Can you work these out from the model? Positions are in its coordinate system, mm. Face numbers are marked on the shaded views. Give positions to 0.01 mm unless a question says otherwise; leave off trailing zeros. Loops run counter-clockwise (first coordinate to the right, second up) from the corner with the lowest first, then second, coordinate; pieces in that order, holes last. Notation, with made-up numbers: (52, 55) -> (88, 55) arc R27 cw to (88, 74) -> close; hole circle Ø3 at (49.5, 34). An arc over 180 degrees is marked (long way). One line per question, with ' | ' between items.
from build123d import *

# Parameters (mm, degrees)
SKETCH1_R           = 39.37
SKETCH1_R_2         = 38.1
BOSS_EXTRUDE1_DEPTH = 685.8
SKETCH2_R           = 1.692869147
CUT_EXTRUDE1_DEPTH  = 61.4
CIRPATTERN3_COUNT   = 3
CUT_EXTRUDE2_DEPTH  = 72.4


with BuildPart() as part:
    # Sketch1 → Boss-Extrude1 (new body)
    with BuildSketch(Plane(origin=(0, 0, 0), x_dir=(1, 0, 0), z_dir=(0, 1, 0))):
        with Locations(Location((0, 0, 0), (0, 0, 270))):
            Circle(SKETCH1_R)
        with Locations(Location((0, 0, 0), (0, 0, 270))):
            Circle(SKETCH1_R_2, mode=Mode.SUBTRACT)
    extrude(amount=BOSS_EXTRUDE1_DEPTH)

    # Sketch2 → Cut-Extrude1 (cut)
    with BuildSketch(Plane.XY):
        with Locations(Location((0, 3.287142885, 0), (0, 0, 90))):
            Circle(SKETCH2_R)
    cut_extrude1 = extrude(amount=-CUT_EXTRUDE1_DEPTH, mode=Mode.SUBTRACT)

    # CirPattern3: Cut-Extrude1 ×3 about axis
    cirpattern3_axis = Axis((0, 0, 0), (0, -1, 0))
    for i in range(1, CIRPATTERN3_COUNT):
        add(cut_extrude1.rotate(cirpattern3_axis, i * 360 / CIRPATTERN3_COUNT), mode=Mode.SUBTRACT)

    # Sketch3 → Cut-Extrude2 (cut)
    with BuildSketch(Plane(origin=(0, 0, 0), x_dir=(0, 0, -1), z_dir=(1, 0, 0))):
        Polygon((-39.37, 513.990392655), (39.37, 513.990392655), (39.37, 282.655028446), (39.37, 269.955028446), (39.37, 263.605028446), (-39.37, 263.605028446), (-39.37, 269.955028446), (-39.37, 276.305028446), (-39.37, 282.655028446), align=None)
    extrude(amount=CUT_EXTRUDE2_DEPTH, mode=Mode.SUBTRACT)


solid = part.part
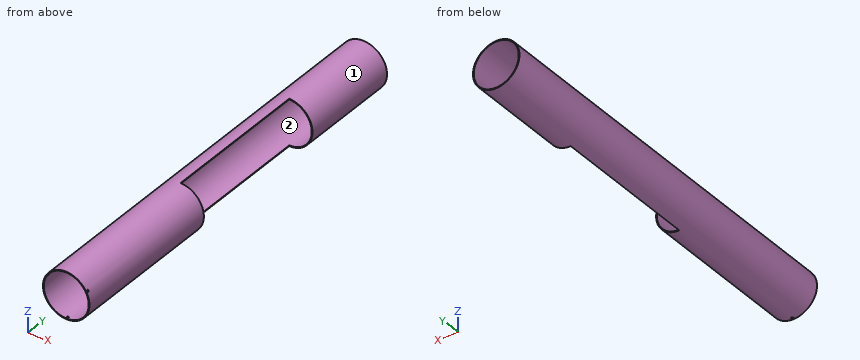
Q1. If we section it at A-A (z = 0): Write out the boundary of the cut face in (x, y), plus the area to 3 significant figures.
Entries:
outline: (-39.37, 0) -> (-38.1, 0) -> (-38.1, 685.8) -> (-39.37, 685.8) -> close; (38.1, 0) -> (39.37, 0) -> (39.37, 263.61) -> (38.1, 263.61) -> close; (38.1, 513.99) -> (39.37, 513.99) -> (39.37, 685.8) -> (38.1, 685.8) -> close | area: 1,420 mm²
Q2. For pin 1 Ø5 at (x, z) = (18.5, 28.5) entering from -Y; pin 2 Ø1.4 at (y, z) = (408, 38.5) entering from +X; pin 3 Ø3 at (y, z) = (507.5, 28.5) entering from -X; pin 4 Ø2 at (x, y) = (0, 3.29) entering from -Z, each with a flat end and sliding along its axis, tell me the tip position at first contact or that it passes through.
Entries:
pin 1: through | pin 2: x = 0 | pin 3: x = -28.65 | pin 4: z = 38.09
Q3. If we section it at D-D (y = 247): Write out the boundary of the cut face in (x, z), plus the area to 3 significant figures.
Entries:
outline: circle Ø78.74 at (0, 0); hole circle Ø76.2 at (0, 0) | area: 309 mm²
Q4. If we section it at B-B (x = -25): Write out the boundary of the cut face in (y, z), plus the area to 3 significant figures.
Entries:
outline: (0, -30.41) -> (685.8, -30.41) -> (685.8, -28.75) -> (0, -28.75) -> close; (0, 28.75) -> (685.8, 28.75) -> (685.8, 30.41) -> (0, 30.41) -> close | area: 2,280 mm²
Q5. If we mould it in two halves opening along X, with no side actions, what happens to the marked faces 1 and 2? For each: pulls with the +X half, pulls with the -X half, needs draft (parallel to the pull), parting line crosses it, or undercut.
Entries:
face 1: parting line crosses it | face 2: undercut
Q6. If I drill on probe 1 along Z at (x, y) = (0, 179); probe 2 along Z at (x, y) = (-20, 656); probe 3 along X at (y, z) = (590, 16), over which ranges is the centre line in solid material (lowest first)? Write a range as from..to.
Entries:
probe 1: -39.37..-38.1, 38.1..39.37 | probe 2: -33.91..-32.43, 32.43..33.91 | probe 3: -35.97..-34.58, 34.58..35.97
Q7. If we section it at C-C (x = 16): Write out the boundary of the cut face in (y, z).
Entries:
outline: (0, -35.97) -> (263.61, -35.97) -> (263.61, -34.58) -> (0, -34.58) -> close; (0, 34.58) -> (263.61, 34.58) -> (263.61, 35.97) -> (0, 35.97) -> close; (513.99, -35.97) -> (685.8, -35.97) -> (685.8, -34.58) -> (513.99, -34.58) -> close; (513.99, 34.58) -> (685.8, 34.58) -> (685.8, 35.97) -> (513.99, 35.97) -> close
